```python
from build123d import *

# Parameters (mm, degrees)
SKETCH1_R               = 1.6
BOSS_EXTRUDE1_DEPTH     = 7.5
SKETCH2_W               = 10
SKETCH2_H               = 6.2
CUT_EXTRUDE1_DEPTH      = 5
CUT_EXTRUDE1_DEPTH_BACK = 5
HOLE1_D                 = 3.7
HOLE1_DEPTH             = 4.4
FILLET1_R               = 2


with BuildPart() as part:
    # Sketch1 → Boss-Extrude1 (new body, symmetric)
    with BuildSketch(Plane.XY):
        with BuildLine():
            Line((-15, 4), (0, 4))
            ThreePointArc((0, 4), (4, 0), (0, -4))
            Line((0, -4), (-15, -4))
            ThreePointArc((-15, -4), (-19, 0), (-15, 4))
        make_face()
        Circle(SKETCH1_R, mode=Mode.SUBTRACT)
        with Locations((-15, 0)):
            Circle(SKETCH1_R, mode=Mode.SUBTRACT)
    extrude(amount=BOSS_EXTRUDE1_DEPTH, both=True)

    # Sketch2 → Cut-Extrude1 (cut, two sides)
    with BuildSketch(Plane(origin=(0, 0, 0), x_dir=(1, 0, 0), z_dir=(0, 1, 0))) as cut_extrude1_sk:
        with Locations((0.5, 0)):
            Rectangle(SKETCH2_W, SKETCH2_H)
        with Locations((-15.5, 0)):
            Rectangle(SKETCH2_W, SKETCH2_H)
    extrude(amount=CUT_EXTRUDE1_DEPTH, mode=Mode.SUBTRACT)
    extrude(cut_extrude1_sk.sketch, amount=-CUT_EXTRUDE1_DEPTH_BACK, mode=Mode.SUBTRACT)

    # Hole1
    with Locations(Plane(origin=(0, 0, -7.5), x_dir=(-1, 0, 0), z_dir=(0, 0, -1))):
        with Locations((0, 0), (15, 0)):
            Hole(HOLE1_D / 2, depth=HOLE1_DEPTH)

    # Fillet1
    fillet1_edges = [part.edges().sort_by_distance(p)[0] for p in [
        (-4.5, -4, 0),
        (-4.5, 4, 0),
        (-10.5, -4, 0),
        (-10.5, 4, 0),
    ]]
    fillet(fillet1_edges, radius=FILLET1_R)


solid = part.part
```
Can you work these out from the model? Positions are in its coordinate system, mm. A direction names the side the tool comes from. Round coordinates to 2 decimals unless told otherwise and drop trailing zeros. Order: outer loops, then holes, each group sorted by start corner. A loop starts at its lowest first (then second) coordinate and runs counter-clockwise, first axis right, second up. Notation, with made-up numbers: (-32, 67) -> (20, 67) arc R23 cw to (20, 90) -> close; hole circle Ø1 at (-40, 66). An arc over 180 degrees is marked (long way). Return JSON: item names as keys, results as strings. Group by question number.
1. If we section it at B-B, the plane y = 0: Write out the boundary of the cut face in (x, z), then the cut area to 3 significant figures.
2. If we section it at C-C, the plane z = 5.25: Write out the boundary of the cut face in (x, y), then the cut area to 3 significant figures.
3. If we section it at A-A, the plane x = -3.5: Write out the boundary of the cut face in (y, z).
4. We'd pull the mould along Z, two halves only. Please class faces 5 (the face through (-7, -4, 0)), 6 (the face through (-7, 0, -7.5)), 7 (the face through (-7, 0, 7.5)), 8 (the face through (-10.5, 0, 0)): released by +Z, released by -Z, zero draft, split by the parting line, or undercut.
5. Will these pins go through, and if not, where does the flat tip stop? pin 1 (3 mm diameter, centred on x = 0, y = 0, fed in from +Z); pin 2 (3 mm diameter, centred on y = 2, z = 1, fed in from -X); pin 3 (3.5 mm diameter, centred on x = 0, y = 0, fed in from -Z); pin 4 (3 mm diameter, centred on y = -0.5, z = -0.5, fed in from +X).
6. I need wall thicknesses on line 1 (Z direction, x = -4, y = 1); line 2 (Y direction, x = -15, z = 4.55); line 3 (X direction, y = -0.5, z = 2.5). Which ranges of each line are inside material? Lowest first, please. Write a range as [from, to].
7. Which directions (+Z, -Z, +X, -X, +Y, -Y) give clear straight access to the entire face, cutting with the end or side of a thin tool? Please do faces 1 (the face through (-4.5, 0, 0)), 2 (the face through (-13.29, -0.71, -5.27)), 3 (the face through (-5.07, -3.4, -0.04)), 4 (the face through (-9.9, 3.43, -0.04)).
8. If we section it at D-D, the plane z = 1: Write out the boundary of the cut face in (x, y).
Output values:
{
 "1": {"outline": "(-19, -7.5) -> (-16.85, -7.5) -> (-16.85, -3.1) -> (-19, -3.1) -> close; (-19, 3.1) -> (-16.6, 3.1) -> (-16.6, 7.5) -> (-19, 7.5) -> close; (-13.4, 3.1) -> (-10.5, 3.1) -> (-10.5, -3.1) -> (-13.15, -3.1) -> (-13.15, -7.5) -> (-1.85, -7.5) -> (-1.85, -3.1) -> (-4.5, -3.1) -> (-4.5, 3.1) -> (-1.6, 3.1) -> (-1.6, 7.5) -> (-13.4, 7.5) -> close; (1.6, 3.1) -> (4, 3.1) -> (4, 7.5) -> (1.6, 7.5) -> close; (1.85, -7.5) -> (4, -7.5) -> (4, -3.1) -> (1.85, -3.1) -> close", "area": "179 mm²"},
 "2": {"outline": "(-15, -4) -> (0, -4) arc R4 ccw to (0, 4) -> (-15, 4) arc R4 ccw to start; hole circle Ø3.2 at (-15, 0); hole circle Ø3.2 at (0, 0)", "area": "154 mm²"},
 "3": {"outline": "(-4, -7.5) -> (4, -7.5) -> (4, -3.1) -> (-4, -3.1) -> close; (-4, 3.1) -> (4, 3.1) -> (4, 7.5) -> (-4, 7.5) -> close"},
 "4": {"face 5": "zero draft", "face 6": "released by -Z", "face 7": "released by +Z", "face 8": "undercut"},
 "5": {"pin 1": "through", "pin 2": "x = -10.5", "pin 3": "z = 3.1", "pin 4": "x = -4.5"},
 "6": {"line 1": "[-7.5, -3.1], [3.1, 7.5]", "line 2": "[-4, -1.6], [1.6, 4]", "line 3": "[-10.5, -4.5]"},
 "7": {"face 1": "+X, +Y, -Y", "face 2": "-Z", "face 3": "+X, -Y", "face 4": "-X, +Y"},
 "8": {"outline": "(-10.5, -2) arc R2 ccw to (-8.5, -4) -> (-6.5, -4) arc R2 ccw to (-4.5, -2) -> (-4.5, 2) arc R2 ccw to (-6.5, 4) -> (-8.5, 4) arc R2 ccw to (-10.5, 2) -> close"}
}
